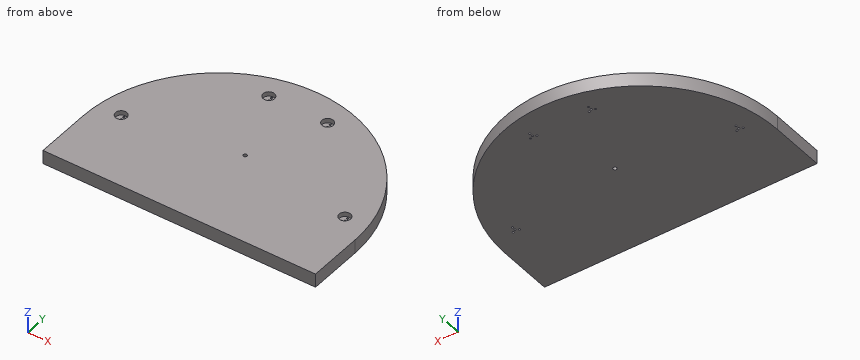
from build123d import *

# Parameters (mm, degrees)
EXTRUDE_1_DEPTH     = 30
SKETCH_2_R          = 12.5
CUT_EXTRUDE_1_DEPTH = 10
SKETCH_4_R          = 2
CUT_EXTRUDE_2_DEPTH = 20
SKETCH_6_R          = 4
CUT_EXTRUDE_3_DEPTH = 59


with BuildPart() as part:
    # 草图1 → 凸台-拉伸1 (new body)
    with BuildSketch(Plane.XY):
        with BuildLine():
            Line((-300, 0), (-300, -120))
            Line((-300, -120), (300, -120))
            Line((300, -120), (300, 0))
            ThreePointArc((300, 0), (0, 300), (-300, 0))
        make_face()
    extrude(amount=EXTRUDE_1_DEPTH)

    # 草图2 → 切除-拉伸1 (cut)
    with BuildSketch(Plane.XY.offset(30)):
        with Locations((-246.201938253, 43.412044417)):
            Circle(SKETCH_2_R)
        with Locations((-64.704761276, 241.481456572)):
            Circle(SKETCH_2_R)
        with Locations(Location((246.201938253, 43.412044417, 0), (0, 0, 180))):
            Circle(SKETCH_2_R)
        with Locations(Location((64.704761276, 241.481456572, 0), (0, 0, 180))):
            Circle(SKETCH_2_R)
    extrude(amount=-CUT_EXTRUDE_1_DEPTH, mode=Mode.SUBTRACT)

    # 草图4 → 切除-拉伸2 (cut)
    with BuildSketch(Plane.XY.offset(20)):
        with Locations((-246.201938253, 43.412044417)):
            Circle(SKETCH_4_R)
        with Locations((-246.201938253, 51.412044417)):
            Circle(SKETCH_4_R)
        with Locations((-253.130141483, 39.412044417)):
            Circle(SKETCH_4_R)
        with Locations((-239.273735023, 39.412044417)):
            Circle(SKETCH_4_R)
        with Locations((-64.704761276, 249.481456572)):
            Circle(SKETCH_4_R)
        with Locations((-71.632964506, 237.481456572)):
            Circle(SKETCH_4_R)
        with Locations((-57.776558045, 237.481456572)):
            Circle(SKETCH_4_R)
        with Locations((-64.704761276, 241.481456572)):
            Circle(SKETCH_4_R)
        with Locations(Location((64.704761276, 241.481456572, 0), (0, 0, 180))):
            Circle(SKETCH_4_R)
        with Locations(Location((57.776558045, 237.481456572, 0), (0, 0, 180))):
            Circle(SKETCH_4_R)
        with Locations(Location((71.632964506, 237.481456572, 0), (0, 0, 180))):
            Circle(SKETCH_4_R)
        with Locations(Location((64.704761276, 249.481456572, 0), (0, 0, 180))):
            Circle(SKETCH_4_R)
        with Locations(Location((239.273735023, 39.412044417, 0), (0, 0, 180))):
            Circle(SKETCH_4_R)
        with Locations(Location((253.130141483, 39.412044417, 0), (0, 0, 180))):
            Circle(SKETCH_4_R)
        with Locations(Location((246.201938253, 51.412044417, 0), (0, 0, 180))):
            Circle(SKETCH_4_R)
        with Locations(Location((246.201938253, 43.412044417, 0), (0, 0, 180))):
            Circle(SKETCH_4_R)
    extrude(amount=-CUT_EXTRUDE_2_DEPTH, mode=Mode.SUBTRACT)

    # 草图6 → 切除-拉伸3 (cut)
    with BuildSketch(Plane(origin=(0, 0, 0), x_dir=(-1, 0, 0), z_dir=(0, 0, -1))):
        with Locations((0, 80)):
            Circle(SKETCH_6_R)
    extrude(amount=-CUT_EXTRUDE_3_DEPTH, mode=Mode.SUBTRACT)


solid = part.part
Check sheet for the modelled part. Datum: model origin and axes. Units: mm. Round coordinates to 2 decimals unless told otherwise and drop trailing zeros. Loops run counter-clockwise (first coordinate to the right, second up) from the corner with the lowest first, then second, coordinate; pieces in that order, holes last.
1. Scan lines: probe 1 along Y at (x, z) = (-65, 10); probe 2 along X at (y, z) = (32, 3); probe 3 along X at (y, z) = (3, 9) (3 decimals). Record each from-to range of solid material in increasing order.
2. Sectioned sample at C-C on x = 100. Record the boundary of the cut face in (y, z).
3. Gauge pin test, flat ends, axial feed: pin 1 Ø1 at (y, z) = (29.5, 23.5) entering from +X; pin 2 Ø12 at (x, z) = (-122, 23.5) entering from +Y; pin 3 Ø1.5 at (x, z) = (76, 11) entering from +Y. Record the tip position at first contact, or that the pin passes through.
4. Sectioned sample at A-A on z = 13.25. Give the number of separate pieces and of enclosed holes in the cut face, and give its area (3 significant figures).
5. Sectioned sample at B-B on x = -176.5. Record the boundary of the cut face in (y, z).
Recorded:
1. probe 1: y = -120 to 239.5, 243.46 to 247.5, 251.46 to 292.87
1. probe 2: x = -298.29 to 298.29
1. probe 3: x = -299.985 to 299.985
2. outline: (-120, 0) - (282.84, 0) - (282.84, 30) - (-120, 30) - close
3. pin 1: stops at x = 298.6
3. pin 2: stops at y = 276.67
3. pin 3: stops at y = 290.41
4. separate pieces: 1
4. enclosed holes: 17
4. area: 213,000 mm2
5. outline: (-120, 0) - (242.59, 0) - (242.59, 30) - (-120, 30) - close
